Verification items for the finished model (mm, model axes). Coordinates: 2 decimals unless noted, no trailing zeros. Order: outer loops, then holes, each group sorted by start corner. A loop starts at its lowest first (then second) coordinate and runs counter-clockwise, first axis right, second up. Notation, with made-up numbers: (17.25, -23.75) -> (73.25, -23.75) arc R35 ccw to (73.25, 11.25) -> close; hole circle Ø3 at (36.25, 23). An arc over 180 degrees is marked (long way). Answer as CSV lines item,"result".
Autodesk Inventor part; units mm, degrees
ref_plane "YZ Plane" through (0, 0, 0) normal (1, 0, 0) x (0, 1, 0)
ref_plane "XZ Plane" through (0, 0, 0) normal (0, 1, 0) x (-1, 0, 0)
ref_plane "XY Plane" through (0, 0, 0) normal (0, 0, 1) x (1, 0, 0)
sketch "スケッチ1" plane through (0, 0, 0) normal (0, 0, 1) x (1, 0, 0)
  line L0 (-106.8804, 63.2098) -> (-114.8803, 63.2581)
  line L1 (-107.2922, -5.024) -> (-115.292, -4.9758)
  line L2 (-4.6996, 92.8548) -> (1.3002, 92.8186)
  line L3 (-5.3383, -12.9733) -> (0.6616, -13.0095)
  line L4 (-79.7382, 110.3105) -> (1.3027, 93.2276)
  line L5 (-88.2817, 72.7187) -> (-79.7382, 110.3105)
  line L6 (-84.055, -53.4485) -> (5.2045, -41.9275)
  line L7 (49.6711, -27.8017) -> (49.6711, -11.6868)
  line L8 (49.6711, -11.6868) -> (84.6711, -11.6868)
  line L9 (5.2045, -41.9275) -> (20.2045, -67.9083)
  line L10 (20.2045, -67.9083) -> (59.6711, -45.1223)
  line L11 (59.6711, -45.1223) -> (49.6711, -27.8017)
  line L12 (-84.055, -53.4485) -> (-90.292, -5.1266)
  circle A0 centre (-111.2619, 0) radius 1.5
  circle A1 centre (-110.9105, 58.2341) radius 1.5
  line L13 (-115.292, -4.9758) -> (-114.8803, 63.2581)
  line L14 (-106.8804, 63.2098) -> (-114.8803, 63.2581)
  line L15 (-106.8804, 63.2098) -> (-107.2922, -5.024)
  line L16 (-107.2922, -5.024) -> (-115.292, -4.9758)
  line L17 (-90.292, -5.1266) -> (-115.292, -4.9758)
  line L18 (-115.292, -4.9758) -> (-114.8803, 63.2581)
  circle A2 centre (-1.7299, 87.8368) radius 1.5
  circle A3 centre (-2.3082, -7.9915) radius 1.5
  line L19 (1.3002, 92.8186) -> (0.6616, -13.0095)
  line L20 (-5.3383, -12.9733) -> (0.6616, -13.0095)
  line L21 (-5.3383, -12.9733) -> (-4.6996, 92.8548)
  line L22 (-4.6996, 92.8548) -> (1.3002, 92.8186)
  line L23 (-114.8803, 63.2581) -> (-4.6996, 92.8548)
  line L24 (1.3002, 92.8186) -> (-4.6996, 92.8548)
  line L25 (1.3002, 92.8186) -> (35.0935, 58.6149)
  line L26 (35.0935, 58.6149) -> (85.0935, 58.3132)
  line L27 (85.0935, 58.3132) -> (84.6711, -11.6868)
  line L28 (-91.5437, -34.2492) -> (2.6068, -22.0969)
  point P0 (0, 0)
  dimension "d25" = 35
  dimension "d27" = 90
  dimension "d29" = 20
  dimension "d30" = 150
  dimension "d31" = 30
  dimension "d60" = 25
  dimension "d61" = 20
  dimension "d62" = 135
  dimension "d63" = 200
  dimension "d64" = 50
  dimension "d65" = 70
extrude "プレート2" add sketch "スケッチ1" along normal blind 2
equation "\"d6\" = Thickness"
equation "\"BendRadius\" = Thickness"
equation "\"BendReliefWidth\" = Thickness"
equation "\"BendReliefDepth\" = 0.5 * Thickness"
equation "\"CornerReliefSize\" = 4 * Thickness"
equation "\"MinimumRemnant\" = 2 * Thickness"
equation "\"TransitionRadius\" = BendRadius"
equation "\"JacobiRadiusSize\" = Thickness"
equation "\"GapSize\" = Thickness"
properties part number "baseframe" material "アルミニウム 6061"
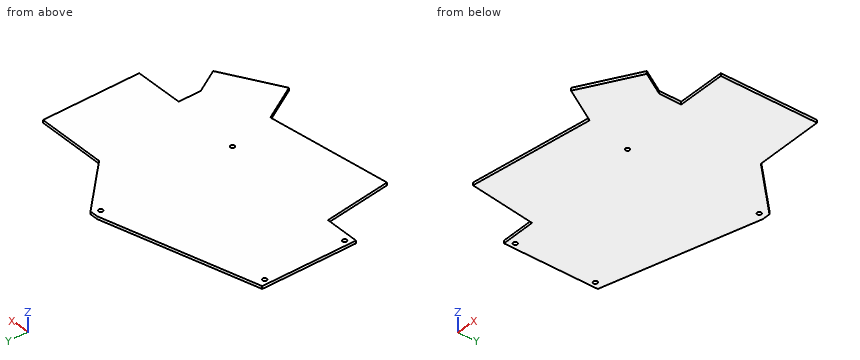
Item 1: Thickness scan on line 1 (Y direction, x = 54, z = 0.7); line 2 (Y direction, x = 24, z = 1); line 3 (Y direction, x = 7.5, z = 0.55). Record the ranges inside material, lowest first.
Answer list:
line 1,"-48.4 to -35.3, -11.69 to 58.5"
line 2,"-65.72 to 69.84"
line 3,"-45.9 to 86.54"
Item 2: Section check B-B, the plane x = -25. Record the boundary of the cut face in (y, z), plus the area to 3 significant figures.
Answer list:
outline,"(-45.83, 0) -> (87.4, 0) -> (87.4, 2) -> (-45.83, 2) -> close"
area,"266 mm2"
Item 3: Depth check by flat-ended pin: pin 1 Ø1 at (y, z) = (-9.5, 0.5) entering from -X; pin 2 Ø1.8 at (x, y) = (-2.31, -7.99) entering from +Z; pin 3 Ø1 at (y, z) = (-43.5, 1) entering from +X. Enter the tip coordinate at first touch or a pass-through.
Answer list:
pin 1,"x = -89.79"
pin 2,"through"
pin 3,"x = 59.02"
Item 4: Section check A-A, the plane z = 1.4. Record the boundary of the cut face in (x, y) (1 decimal), plus the area to 3 significant figures.
Answer list:
outline,"(-115.3, -5) -> (-107.3, -5) -> (-90.3, -5.1) -> (-84.1, -53.4) -> (5.2, -41.9) -> (20.2, -67.9) -> (59.7, -45.1) -> (49.7, -27.8) -> (49.7, -11.7) -> (84.7, -11.7) -> (85.1, 58.3) -> (35.1, 58.6) -> (1.3, 92.8) -> (-4.7, 92.9) -> (-114.9, 63.3) -> close; hole circle Ø3 at (-111.3, 0); hole circle Ø3 at (-110.9, 58.2); hole circle Ø3 at (-2.3, -8); hole circle Ø3 at (-1.7, 87.8)"
area,"22,300 mm2"
Item 5: Section check C-C, the plane y = 78. Record the boundary of the cut face in (x, z), plus the area to 3 significant figures.
Answer list:
outline,"(-60, 0) -> (15.94, 0) -> (15.94, 2) -> (-60, 2) -> close"
area,"152 mm2"
